from build123d import *

# Parameters (mm, degrees)
BOSS_EXTRUDE1_DEPTH = 102
SKETCH5_R           = 13
BOSS_EXTRUDE2_DEPTH = 2.5
BOSS_EXTRUDE3_DEPTH = 1
FILLET1_R           = 1


with BuildPart() as part:
    # Sketch1 → Revolve1 (revolve)
    with BuildSketch(Plane.XY, mode=Mode.PRIVATE) as revolve1_sk:
        Polygon((0, 0), (7.5, 0), (7.5, 3), (6, 3), (6, 5), (10, 5), (10, 6), (0, 6), align=None)
    revolve(revolve1_sk.sketch.rotate(Axis((0, 6, 0), (0, -1, 0)), 180), axis=Axis((0, 6, 0), (0, -1, 0)))

    # Sketch4 → Boss-Extrude1 (add)
    with BuildSketch(Plane(origin=(0, 6, 0), x_dir=(1, 0, 0), z_dir=(0, 1, 0))):
        with BuildLine():
            Line((-1, 8), (-1, 1.5))
            ThreePointArc((-1, 1.5), (-1.146446609, 1.146446609), (-1.5, 1))
            Line((-1.5, 1), (-8, 1))
            ThreePointArc((-8, 1), (-9, 0), (-8, -1))
            Line((-8, -1), (-1.5, -1))
            ThreePointArc((-1.5, -1), (-1.146446609, -1.146446609), (-1, -1.5))
            Line((-1, -1.5), (-1, -8))
            ThreePointArc((-1, -8), (0, -9), (1, -8))
            Line((1, -8), (1, -1.5))
            ThreePointArc((1, -1.5), (1.146446609, -1.146446609), (1.5, -1))
            Line((1.5, -1), (8, -1))
            ThreePointArc((8, -1), (9, 0), (8, 1))
            Line((8, 1), (1.5, 1))
            ThreePointArc((1.5, 1), (1.146446609, 1.146446609), (1, 1.5))
            Line((1, 1.5), (1, 8))
            ThreePointArc((1, 8), (0, 9), (-1, 8))
        make_face()
    extrude(amount=BOSS_EXTRUDE1_DEPTH)

    # Sketch5 → Boss-Extrude2 (add)
    with BuildSketch(Plane(origin=(0, 108, 0), x_dir=(1, 0, 0), z_dir=(0, 1, 0))):
        with Locations(Location((0, 0, 0), (0, 0, 180))):
            Circle(SKETCH5_R)
    extrude(amount=BOSS_EXTRUDE2_DEPTH)

    # Sketch6 → Boss-Extrude3 (add)
    with BuildSketch(Plane(origin=(0, 110.5, 0), x_dir=(1, 0, 0), z_dir=(0, 1, 0))):
        with BuildLine():
            Line((-1.5, 10), (-1.5, -10))
            ThreePointArc((-1.5, -10), (0, -11.5), (1.5, -10))
            Line((1.5, -10), (1.5, 10))
            ThreePointArc((1.5, 10), (0, 11.5), (-1.5, 10))
        make_face()
        with BuildLine():
            Line((-5.7, 8), (-5.7, -7.799265344))
            ThreePointArc((-5.7, -7.799265344), (-4.2, -9.299265344), (-2.7, -7.799265344))
            Line((-2.7, -7.799265344), (-2.7, 8))
            ThreePointArc((-2.7, 8), (-4.2, 9.5), (-5.7, 8))
        make_face()
        with BuildLine():
            Line((-9.9, 6), (-9.9, -6.275084591))
            ThreePointArc((-9.9, -6.275084591), (-8.4, -7.775084591), (-6.9, -6.275084591))
            Line((-6.9, -6.275084591), (-6.9, 6))
            ThreePointArc((-6.9, 6), (-8.4, 7.5), (-9.9, 6))
        make_face()
        with BuildLine():
            Line((9.9, 6), (9.9, -6.275084591))
            ThreePointArc((9.9, -6.275084591), (8.4, -7.775084591), (6.9, -6.275084591))
            Line((6.9, -6.275084591), (6.9, 6))
            ThreePointArc((6.9, 6), (8.4, 7.5), (9.9, 6))
        make_face()
        with BuildLine():
            Line((5.7, 8), (5.7, -7.799265344))
            ThreePointArc((5.7, -7.799265344), (4.2, -9.299265344), (2.7, -7.799265344))
            Line((2.7, -7.799265344), (2.7, 8))
            ThreePointArc((2.7, 8), (4.2, 9.5), (5.7, 8))
        make_face()
    extrude(amount=BOSS_EXTRUDE3_DEPTH)

    # Fillet1
    fillet1_edges = [part.edges().sort_by_distance(p)[0] for p in [
        (9.9, 111.5, 0.137542295),
        (8.4, 111.5, 7.775084591),
        (6.9, 111.5, 0.137542295),
        (8.4, 111.5, -7.5),
        (5.7, 111.5, -0.100367328),
        (4.2, 111.5, 9.299265344),
        (2.7, 111.5, -0.100367328),
        (4.2, 111.5, -9.5),
        (1.5, 111.5, 0),
        (0, 111.5, 11.5),
        (-1.5, 111.5, 0),
        (0, 111.5, -11.5),
        (-2.7, 111.5, -0.100367328),
        (-4.2, 111.5, 9.299265344),
        (-5.7, 111.5, -0.100367328),
        (-4.2, 111.5, -9.5),
        (-6.9, 111.5, 0.137542295),
        (-8.4, 111.5, 7.775084591),
        (-9.9, 111.5, 0.137542295),
        (-8.4, 111.5, -7.5),
    ]]
    fillet(fillet1_edges, radius=FILLET1_R - 0.0001)  # a hair under: the kernel refuses the full size


solid = part.part
The listing builds one solid part. Answer for the finished solid, in the listing's coordinates (mm). A direction names the side the tool comes from. Give positions to 0.01 mm unless a question says otherwise; leave off trailing zeros. Write each loop counter-clockwise with the first axis right and the second up, starting at its lowest first coordinate (ties: lowest second). Pieces come first, ordered by that corner, then holes.
Item 1: Determine the mould class of faces 6 (the flat face through (-1, 56, -5)), 7 (the flat face through (1, 56, 5)), 8 (the flat face through (6, 110.5, 0)), 9 (the flat face through (5, 56, -1)) for opening direction X: released by +X, released by -X, zero draft, split by the parting line, or undercut.
Item 2: Which of the six approach directions +Z, -Z, +X, -X, +Y, -Y give full straight-line access (tool end or side, diameter ignored) to faces 1 (the flat face through (-2, 6, 2)), 2 (the cylindrical face through (9, 56, 0)), 3 (the cylindrical face through (-4.032, 1.521, -6.324)), 4 (the cylindrical face through (-9, 56, 0)), 5 (the flat face through (-5, 56, 1))?
Item 3: Find the intervals of material crossed by line 1 along Y through (x, z) = (6, -7.5); line 2 along Y through (x, z) = (2.25, -3.75); line 3 along Y through (x, z) = (-7, 8), in increasing order.
Item 4: Section A-A, the plane y = 96 is taken. Write down the section's boundary in (x, z).
Item 5: Flat-ended cylindrical pins translate along their axes: P1, Ø1.5, axis at y = 100, z = -8.5, coming from the -X side; P2, Ø3, axis at y = 81.5, z = -4, coming from the +X side; P3, Ø1.5, axis at x = -9.5, y = 89, coming from the +Z side. Find the tip coordinate at first contact, or state that the pin passes through.
Completed:
1. face 6: released by -X
1. face 7: released by +X
1. face 8: undercut
1. face 9: zero draft
2. face 1: none
2. face 2: +X
2. face 3: -Y
2. face 4: -X
2. face 5: +Z, -X
3. line 1: y = 5 to 6, 108 to 110.5
3. line 2: y = 0 to 6, 108 to 110.5
3. line 3: y = 108 to 110.5
4. outline: (-8, -1) - (-1.5, -1) arc R0.5 cw to (-1, -1.5) - (-1, -8) arc R1 ccw to (1, -8) - (1, -1.5) arc R0.5 cw to (1.5, -1) - (8, -1) arc R1 ccw to (8, 1) - (1.5, 1) arc R0.5 cw to (1, 1.5) - (1, 8) arc R1 ccw to (-1, 8) - (-1, 1.5) arc R0.5 cw to (-1.5, 1) - (-8, 1) arc R1 ccw to start
5. P1: stops at x = -1
5. P2: stops at x = 1
5. P3: stops at z = 0.66
